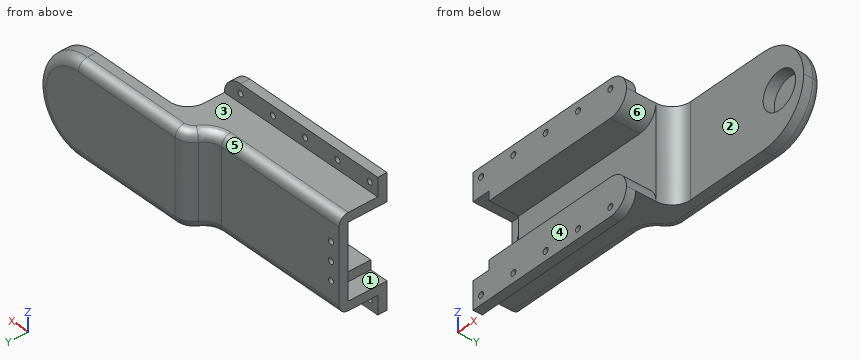
Autodesk Inventor part; units mm, degrees
ref_plane "YZ Plane" through (0, 0, 0) normal (1, 0, 0) x (0, 1, 0)
ref_plane "XZ Plane" through (0, 0, 0) normal (0, 1, 0) x (-1, 0, 0)
ref_plane "XY Plane" through (0, 0, 0) normal (0, 0, 1) x (1, 0, 0)
sketch "Sketch1" plane through (0, 0, 0) normal (0, 0, 1) x (1, 0, 0)
  line L0 (-87.5, -18) -> (87.5, -18)
  line L1 (87.5, -18) -> (87.5, 18)
  line L2 (87.5, 18) -> (-87.5, 18)
  line L3 (-87.5, 18) -> (-87.5, -18)
  line L4 (-87.5, -18) -> (87.5, 18) construction
  line L5 (87.5, -18) -> (-87.5, 18) construction
  line L6 (-87.5, 18) -> (-7.5, 18)
  line L7 (-7.5, 18) -> (-7.5, 8)
  line L8 (-7.5, 8) -> (-87.5, 8)
  line L9 (-87.5, 8) -> (-87.5, 18)
  line L10 (87.5, -18) -> (7.5, -18)
  line L11 (7.5, -18) -> (7.5, 8)
  line L12 (7.5, 8) -> (87.5, 8)
  line L13 (87.5, 8) -> (87.5, -18)
  point P0 (0, 0)
  point P1 (87.5, 8)
  point P2 (-7.5, 18)
  point P3 (7.5, -18)
  point P4 (72.5, 8)
  dimension "d1" = 36
  dimension "d2" = 80
  dimension "d3" = 10
  dimension "d4" = 80
  dimension "d5" = 26
  dimension "d62" = 15
  dimension "d63" = 160
extrude "Extrusion1" add sketch "Sketch1" along normal blind 50 contours L3 L8 L7 L2 L1 L12 L11 L0
fillet "Fillet1" radius 10 3 edges at (-7.5, 18, 25) (-7.5, 8, 25) (7.5, 8, 25)
sketch "Sketch2" plane through (-87.5, -18, 0) normal (-1, 0, 0) x (0, 0, 1)
  line L0 (10, 0) -> (40, 0)
  line L1 (40, 0) -> (40, 16)
  line L2 (40, 16) -> (10, 16)
  line L3 (10, 16) -> (10, 0)
  line L4 (0, 26) -> (0, 0)
  line L5 (50, 26) -> (50, 0)
  line L6 (0, 0) -> (50, 0)
  line L7 (0, 26) -> (50, 26)
  point P0 (0, 18)
  dimension "d9" = 10
  dimension "d10" = 10
  dimension "d11" = 10
extrude "Extrusion2" cut sketch "Sketch2" against normal through all contours L3 L2 L1 L0
sketch "Sketch3" plane through (87.5, 8, 0) normal (0, -1, 0) x (1, 0, 0)
  circle A0 centre (-15, 25) radius 10.05
  line L0 (0, 0) -> (0, 50)
  circle A1 centre (-15, 25) radius 15
  point P0 (-87.5, 0)
  point P1 (0, 25)
  dimension "d14" = 20.1
  dimension "d15" = 30
extrude "Extrusion3" cut sketch "Sketch3" against normal blind 6 contours A0
sketch "Sketch4" plane through (-87.5, -18, 0) normal (0, -1, 0) x (1, 0, 0)
  line L0 (0, 50) -> (95, 50)
  line L1 (0, 50) -> (95, 50)
  line L2 (95, 50) -> (95, 60)
  line L3 (95, 60) -> (0, 60)
  line L4 (0, 60) -> (0, 50)
  line L5 (95, 40) -> (95, 50)
  line L6 (0, 0) -> (0, 50)
  line L7 (0, 25) -> (90, 25)
  circle A0 centre (5, 55) radius 1.55
  circle A1 centre (25, 55) radius 1.55
  circle A2 centre (45, 55) radius 1.55
  circle A3 centre (65, 55) radius 1.55
  circle A4 centre (85, 55) radius 1.55
  line L8 (0, 0) -> (95, 0)
  line L9 (0, 0) -> (95, 0)
  line L10 (95, 0) -> (95, -10)
  line L11 (95, -10) -> (0, -10)
  line L12 (0, -10) -> (0, 0)
  circle A5 centre (5, -5) radius 1.55
  circle A6 centre (25, -5) radius 1.55
  circle A7 centre (45, -5) radius 1.55
  circle A8 centre (65, -5) radius 1.55
  circle A9 centre (85, -5) radius 1.55
  line L13 (0, 0) -> (95, 0)
  line L14 (0, 0) -> (95, 0)
  line L15 (95, 0) -> (95, -10)
  line L16 (95, -10) -> (0, -10)
  line L17 (0, -10) -> (0, 0)
  circle A10 centre (5, -5) radius 1.55
  circle A11 centre (25, -5) radius 1.55
  circle A12 centre (45, -5) radius 1.55
  circle A13 centre (65, -5) radius 1.55
  circle A14 centre (85, -5) radius 1.55
  point P0 (87.5, 0)
  point P1 (0, 55)
  point P2 (0, -5)
  dimension "d18" = 10
  dimension "d19" = 3.1
  dimension "d20" = 5
  dimension "d23" = 20
extrude "Extrusion4" add sketch "Sketch4" against normal blind 5
sketch "Sketch9" plane through (-87.5, 8, 0) normal (-1, 0, 0) x (0, 0, 1)
  line L0 (4.9, -26) -> (45.1, -26)
  line L1 (45.1, -26) -> (45.1, -4.9)
  line L2 (45.1, -4.9) -> (4.9, -4.9)
  line L3 (4.9, -4.9) -> (4.9, -26)
  line L4 (40, -26) -> (60, -26)
  line L5 (10, -26) -> (10, -10)
  line L6 (40, -10) -> (40, -26)
  line L7 (10, -10) -> (40, -10)
  point P0 (0, -8)
  point P1 (40, -26)
  dimension "d44" = 5.1
  dimension "d45" = 5.1
  dimension "d46" = 5.1
extrude "Extrusion7" cut sketch "Sketch9" against normal blind 10 contours L3 L2 L1 L0 L6 L7 L5
sketch "Sketch11" plane through (-87.5, 3.1, 4.9) normal (0, -1, 0) x (1, 0, 0)
  circle A0 centre (5, 10) radius 1.55
  line L0 (10, 0) -> (0, 0)
  line L1 (0, 40.2) -> (10, 40.2)
  line L2 (10, 0) -> (10, 40.2)
  circle A1 centre (5, 20) radius 1.55
  circle A2 centre (5, 30) radius 1.55
  point P0 (87.5, -4.9)
  point P1 (5, 0)
  dimension "d50" = 3.1
  dimension "d51" = 10
  dimension "d54" = 10
fillet "Fillet2" radius 25 2 edges at (87.5, 13, 50) (87.5, 13, 0)
extrude "Extrusion8" cut sketch "Sketch11" against normal blind 10
fillet "Fillet3" radius 10 2 edges at (7.5, -15.5, 60) (7.5, -15.5, -10)
fillet "Fillet4" radius 5 9 edges at (-2.5006, 16.6603, 50) (-9.8208, 9.3398, 50) (-51.1605, 8, 50) (80.1778, 18, 42.6778) (32.4997, 18, 0) (-2.5006, 16.6603, 0) (-9.8208, 9.3398, 0) (-51.1605, 8, 0) (32.4997, 18, 50)
fillet "Fillet6" radius 10 2 edges at (7.5, -10, 10) (7.5, -10, 40)
equation "\"screw_out_width\" = 7.5"
properties part number "pulley_case_part_2_v2"
The model under review builds one solid part; all positions refer to its coordinate system, in mm. Face numbers are marked on the shaded views. A direction names the side the tool comes from. Give positions to 0.01 mm unless a question says otherwise; leave off trailing zeros. Write each loop counter-clockwise with the first axis right and the second up, starting at its lowest first coordinate (ties: lowest second). Pieces come first, ordered by that corner, then holes. Notation, with made-up numbers: M 16,44 L 27,44 A14 cw 27,59 Z; hole C 3,19.5 d3. An arc over 180 degrees is marked long. Write item = value, one per line. Start each with the question number.
Q1. We need section D-D (x = -16.5). State the section outline as (y, z) points.
Q2. We need section A-A (x = -42.5). State the section outline as (y, z) points, plus the area to 3 significant figures.
Q3. We need section C-C (z = -5). State the section outline as (x, y) points, plus the area to 3 significant figures.
Q4. Mouldability with a two-part tool opening along Z and no side actions: class the marked faces 4, 5 and 6 as released by +Z, released by -Z, zero draft, split by the parting line, or undercut.
Q5. For line 1 (Z direction, x = -62.5, y = -14.7); line 2 (Z direction, x = -82.5, y = -15.35); line 3 (Y direction, x = 43, z = 7.5), list the stretches that pass through material, from the lowest coordinate up.
Q6. Clearance check with flat-ended pins moving along their axes: pin 1 (1.5 mm diameter, centred on x = -34, z = 26.5, fed in from -Y); pin 2 (3 mm diameter, centred on x = -2.5, z = -5, fed in from +Y); pin 3 (22 mm diameter, centred on x = 77, z = 22.5, fed in from -Y); pin 4 (10 mm diameter, centred on x = -2, y = 0, fed in from -Z). State where each tip first meets the part, or that it passes through.
Q7. Machinability: for the marked faces 1, 2 and 3, which of the approach directions +Z, -Z, +X, -X, +Y, -Y give a long, thin tool a straight path to every point of the face, cutting with its end or side? Answer none if there is none.
Result set:
q1.outline = M -18,-10 L -13,-10 L -13,0 L 3,0 A5 ccw 8,5 L 8,45 A5 ccw 3,50 L -13,50 L -13,60 L -18,60 L -18,40 L -2,40 L -2,10 L -18,10 Z
q2.outline = M -18,-10 L -13,-10 L -13,-6.55 L -18,-6.55 Z; M -18,-3.45 L -13,-3.45 L -13,0 L 3,0 A5 ccw 8,5 L 8,45 A5 ccw 3,50 L -13,50 L -13,53.45 L -18,53.45 L -18,40 L -2,40 L -2,10 L -18,10 Z; M -18,56.55 L -13,56.55 L -13,60 L -18,60 Z
q2.area = 878 mm2
q3.outline = M -87.5,-18 L -84.05,-18 L -84.05,-13 L -87.5,-13 Z; M -80.95,-18 L -64.05,-18 L -64.05,-13 L -80.95,-13 Z; M -60.95,-18 L -44.05,-18 L -44.05,-13 L -60.95,-13 Z; M -40.95,-18 L -24.05,-18 L -24.05,-13 L -40.95,-13 Z; M -20.95,-18 L -4.05,-18 L -4.05,-13 L -20.95,-13 Z; M -0.95,-18 L 6.16,-18 L 6.16,-13 L -0.95,-13 Z
q3.area = 391 mm2
q4.face_4 = zero draft
q4.face_5 = released by +Z
q4.face_6 = undercut
q5.line_1 = -10 to -6.55, -3.45 to 10, 40 to 53.45, 56.55 to 60
q5.line_2 = -10 to -6.55, -3.45 to 4.9, 45.1 to 53.45, 56.55 to 60
q5.line_3 = 8 to 18
q6.pin_1 = -2
q6.pin_2 = through
q6.pin_3 = 8
q6.pin_4 = 0
q7.face_1 = -X, -Y
q7.face_2 = +Z, -Z, +X, -Y
q7.face_3 = +Z, +X, -X, +Y
